Input: part model. Units: mm. Frame: model coordinates. Face numbers are marked on the shaded views. A direction names the side the tool comes from. Coordinates: 2 decimals unless noted, no trailing zeros. Loops run counter-clockwise (first coordinate to the right, second up) from the corner with the lowest first, then second, coordinate; pieces in that order, holes last. Notation, with made-up numbers: (57, 6) -> (88, 6) arc R21 cw to (88, 37) -> close; hole circle Ø1 at (3, 13.25). An arc over 180 degrees is marked (long way). Answer as a JSON object with one key per item and string values.
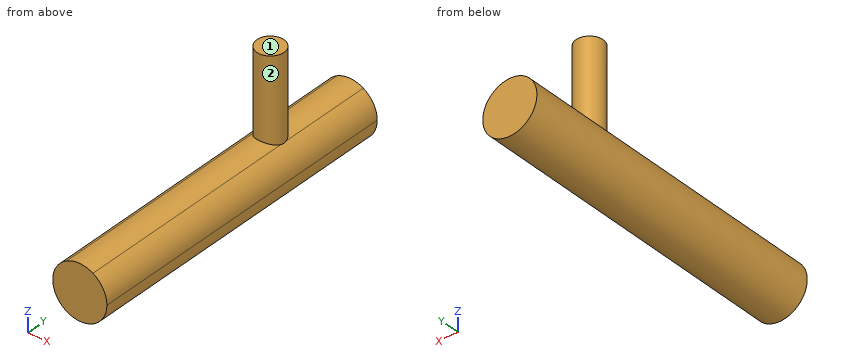
from build123d import *
from build123d import SkipClean  # not in build123d's __all__

# Parameters (mm, degrees)
F1_DEPTH = 76.2
F2_R     = 3.175
F3_DEPTH = 25.4


with BuildPart() as f1:
    # F0 (on Front) → F1 (new body)
    with BuildSketch(Plane.XZ):
        with BuildLine():
            ThreePointArc((-3.0741805311, 5.55625), (-3.2250157851, -5.4700798153), (6.35, 0))
            ThreePointArc((6.35, 0), (5.4700798153, 3.2250157851), (3.0741805311, 5.55625))
            ThreePointArc((3.0741805311, 5.55625), (0, 6.35), (-3.0741805311, 5.55625))
        make_face()
    extrude(amount=F1_DEPTH)

    # F2 (on Top) → F3 (join)
    with BuildSketch(Plane.XY):
        with Locations((0, -22.4732574466)):
            Circle(F2_R)
    with SkipClean():  # cleaning this boolean's faces spoils the solid; the shape is the same uncleaned
        extrude(amount=F3_DEPTH)


solid = f1.part
1. Section query A-A (x = 0). Return loops of the section in (y, z), plus the area to 3 significant figures.
Reply:
{"outline": "(-76.2, -6.35) -> (0, -6.35) -> (0, 6.35) -> (-19.3, 6.35) -> (-19.3, 25.4) -> (-25.65, 25.4) -> (-25.65, 6.35) -> (-76.2, 6.35) -> close", "area": "1,090 mm2"}
2. Access query for the marked faces 1 and 2. Directions: +Z, -Z, +X, -X, +Y, -Y. A direction counts if a zero-diameter tool reaches every point of the face in a straight line with its end or side. Return the directions, or none.
Reply:
{"face 1": "+Z, +X, -X, +Y, -Y", "face 2": "+Z"}
3. Section query C-C (z = -1.5). Return loops of the section in (x, y).
Reply:
{"outline": "(-6.17, -76.2) -> (6.17, -76.2) -> (6.17, 0) -> (-6.17, 0) -> close"}
4. Section query B-B (y = -70). Return loops of the section in (x, z).
Reply:
{"outline": "circle Ø12.7 at (0, 0)"}
5. Line query: line 1 along Z through (x, y) = (-5.5, -10.5); line 2 along Z through (x, y) = (0, -37); line 3 along X through (y, z) = (-16, 4). Output: solid intervals per line, ascending.
Reply:
{"line 1": "z = -3.17 to 3.17", "line 2": "z = -6.35 to 6.35", "line 3": "x = -4.93 to 4.93"}
6. Pin query (flat end, axial travel): P1, Ø2, axis at x = -4.5, z = 10.5, coming from the +Y side; P2, Ø3, axis at x = 1.5, y = -33.5, coming from the +Z side; P3, Ø2, axis at x = -2.5, z = 14.5, coming from the -Y side; P4, Ø8, axis at y = -31.5, z = 5.5, coming from the +X side. Return the tip coordinate at first contact, or that it passes through.
Reply:
{"P1": "passes through", "P2": "stops at z = 6.35", "P3": "stops at y = -25.27", "P4": "stops at x = 6.17"}
